Autodesk Inventor part; units mm, degrees
ref_plane "YZ Plane" through (0, 0, 0) normal (1, 0, 0) x (0, 1, 0)
ref_plane "XZ Plane" through (0, 0, 0) normal (0, 1, 0) x (-1, 0, 0)
sketch "Sketch1" plane through (0, 0, 0) normal (0, 0, 1) x (1, 0, 0)
  circle A0 centre (0, 0) radius 6.35
  dimension "d0" = 12.7
extrude "Extrusion1" add sketch "Sketch1" along normal mid plane 203.2
ref_plane "Work Plane1" through (0, 0, 81.7626) normal (0, 0, 1) x (1, 0, 0)
sketch "Sketch2" plane through (0, 0, 81.7626) normal (0, 0, 1) x (1, 0, 0)
  circle A0 centre (0, 0) radius 6.35
  circle A1 centre (0, 0) radius 6.35
  circle A2 centre (0, 0) radius 5.9436
  dimension "d4" = 12.7
  dimension "d5" = 11.8872
extrude "Extrusion2" cut sketch "Sketch2" against normal blind 0.9906
mirror "Mirror1" about plane through (0, 0, 0) normal (0, 0, 1) of "Extrusion2"
ref_plane "Work Plane3" through (0, 0, 45.4914) normal (0, 0, 1) x (1, 0, 0)
sketch "Sketch3" plane through (0, 0, 45.4914) normal (0, 0, 1) x (1, 0, 0)
  circle A0 centre (0, 0) radius 6.35
  circle A1 centre (0, 0) radius 6.35
  circle A2 centre (0, 0) radius 5.9436
  dimension "d9" = 12.7
  dimension "d10" = 11.8872
extrude "Extrusion3" cut sketch "Sketch3" along normal blind 0.9906
mirror "Mirror2" about plane through (0, 0, 0) normal (0, 0, 1) of "Extrusion3"
ref_plane "Work Plane2" through (0, 0, -81.7626) normal (0, 0, 1) x (1, 0, 0)
ref_plane "Work Plane4" through (0, 0, -45.4914) normal (0, 0, 1) x (1, 0, 0)
properties part number "Boom to Stick .5in. Pin" material "Aluminum 6061"
CAD build for the part. Positions are in the model's coordinates, mm. A direction names the side the tool comes from. Give positions to 0.01 mm unless a question says otherwise; leave off trailing zeros. Write each loop counter-clockwise with the first axis right and the second up, starting at its lowest first coordinate (ties: lowest second). Pieces come first, ordered by that corner, then holes. Notation, with made-up numbers: M -40,-32.75 L 17,-32.75 A27 ccw 17,-16.75 Z; hole C -18.75,72.25 d8. An arc over 180 degrees is marked long. Return JSON: item names as keys, results as strings. Group by question number.
(1) Flat gauge pins, fed straight in: pin 1 Ø1.5 at (y, z) = (-2, -78) entering from -X; pin 2 Ø5 at (y, z) = (4.5, 68) entering from +X; pin 3 Ø1 at (x, z) = (-2.5, 58) entering from +Y. Where does each tip first touch, or does it go through?
(2) Drill centre lines: L1, parallel to Z at x = 5.5, y = -2.5; L2, parallel to Y at x = -2.25, z = 82; L3, parallel to X at y = 2, z = -41.5. Where is each one in solid material? Low to high. Write a range as [from, to].
(3) 3-axis set-ups, long thin cutter, end or side, ignore diameter. For faces 1 (the face through (-1.38, 6.2, -63.87)), 2 (the face through (5.669, 1.785, 81.274)): which of +Z, -Z, +X, -X, +Y, -Y reach the whole face in a straight line?
(4) Mould opens along Z. For faces 3 (the face through (0, 0, 101.6)), 4 (the face through (5.669, 1.785, -45.98)), 5 (the face through (-1.38, 6.2, -0.64)) say: pulls with the +Z half, pulls with the -Z half, needs draft (parallel to the pull), parting line crosses it, or undercut.
(5) Band-saw the part on A-A (z = -31.5). Give the cut face in (x, y), and give its area (3 significant figures).
Entries:
{
 "1": {"pin 1": "stops at x = -6.23", "pin 2": "stops at x = 6.03", "pin 3": "stops at y = 6.03"},
 "2": {"L1": "z = [-101.6, -81.76], [-80.77, -46.48], [-45.49, 45.49], [46.48, 80.77], [81.76, 101.6]", "L2": "y = [-5.94, 5.94]", "L3": "x = [-6.03, 6.03]"},
 "3": {"face 1": "+Z, -Z", "face 2": "none"},
 "4": {"face 3": "pulls with the +Z half", "face 4": "undercut", "face 5": "needs draft"},
 "5": {"outline": "C 0,0 d12.7", "area": "127 mm^2"}
}
